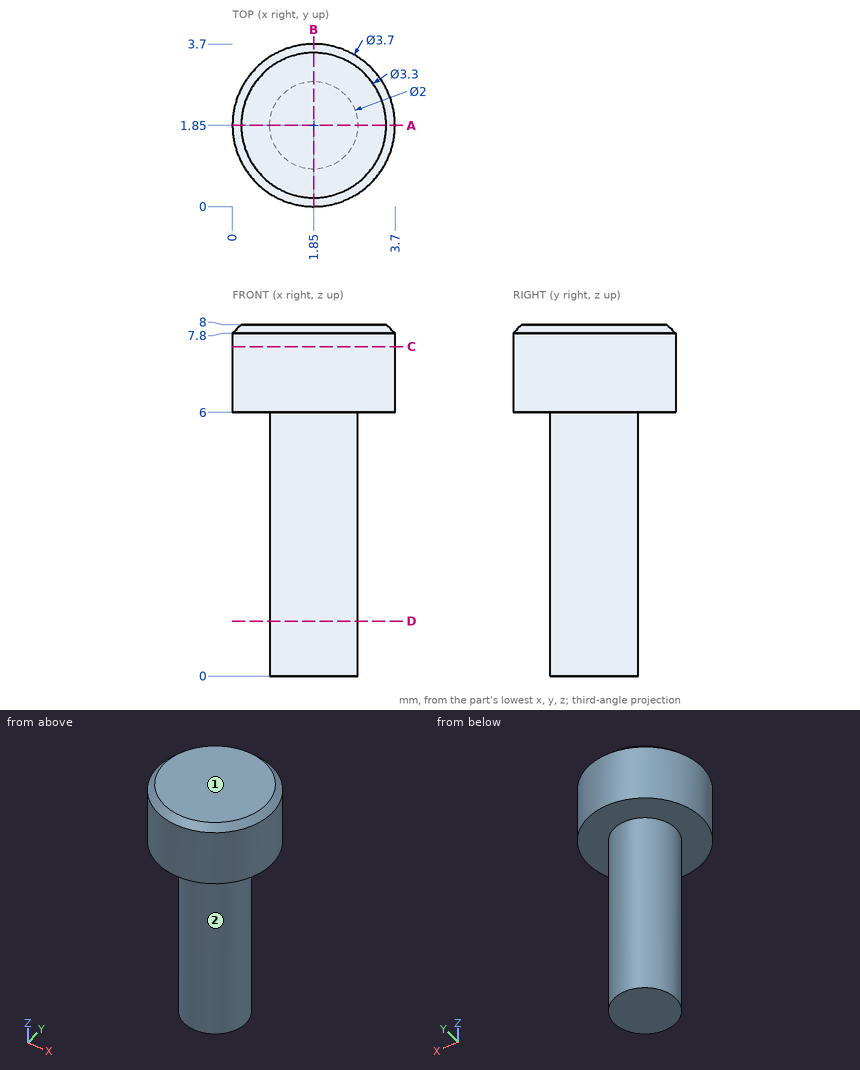
Source: three-view drawing plus pictorial views. Frame: mm from the lowest corner of the part. A direction names the side the tool comes from. Give positions to 0.01 mm unless a question says otherwise; leave off trailing zeros. Loops run counter-clockwise (first coordinate to the right, second up) from the corner with the lowest first, then second, coordinate; pieces in that order, holes last.
1) Line query: L1, parallel to Z at x = 2.4, y = 0.5; L2, parallel to X at y = 1.9, z = 5.75; L3, parallel to Y at x = 3.5, z = 6.5. Output: solid intervals per line, ascending.
A:
L1: z = 6 to 8
L2: x = 0.85 to 2.85
L3: y = 1.01 to 2.69
2) Section query C-C on z = 7.5. Return the cut outline in (x, y), and give its area (3 significant figures).
A:
outline: circle Ø3.7 at (1.85, 1.85)
area: 10.8 mm2
3) Contact query for flat-ended pins moving along their axis: pin 1 (1.5 mm diameter, centred on y = 0.5, z = 4.5, fed in from -X); pin 2 (1.5 mm diameter, centred on x = 3, z = 2, fed in from +Y). Output: stop coordinate, or through.
A:
pin 1: stops at x = 1.05
pin 2: stops at y = 2.77
4) Reachability of the marked faces 1 and 2 from +Z, -Z, +X, -X, +Y, -Y: full face, straight path, thin tool, end or side. Return the list, or none.
A:
face 1: +Z, +X, -X, +Y, -Y
face 2: -Z
5) Section query A-A on y = 1.85. Return the cut outline in (x, z), and give its area (3 significant figures).
A:
outline: (0, 6) - (0.85, 6) - (0.85, 0) - (2.85, 0) - (2.85, 6) - (3.7, 6) - (3.7, 7.8) - (3.5, 8) - (0.2, 8) - (0, 7.8) - close
area: 19.4 mm2
6) Section query D-D on z = 1.25. Return the cut outline in (x, y).
A:
outline: circle Ø2 at (1.85, 1.85)
